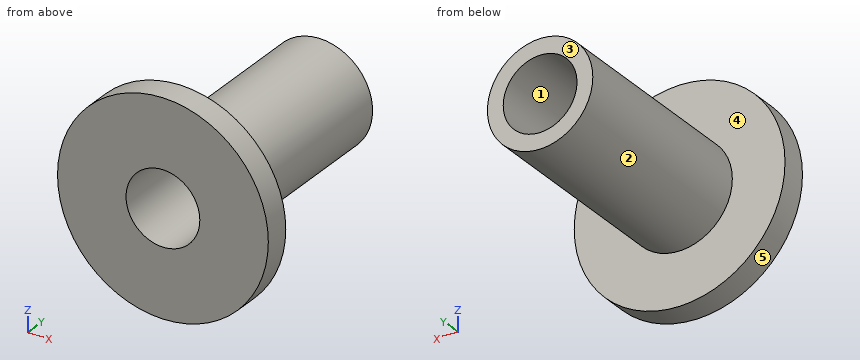
Autodesk Inventor part; units mm, degrees
ref_plane "YZ Plane" through (0, 0, 0) normal (1, 0, 0) x (0, 1, 0)
ref_plane "XZ Plane" through (0, 0, 0) normal (0, 1, 0) x (-1, 0, 0)
ref_plane "XY Plane" through (0, 0, 0) normal (0, 0, 1) x (1, 0, 0)
sketch "Sketch1" plane through (0, 0, 0) normal (0, 1, 0) x (-1, 0, 0)
  circle A0 centre (0, 0) radius 6.35
  dimension "d0" = 12.7
extrude "Extrusion1" add sketch "Sketch1" along normal blind 25.4
sketch "Sketch2" plane through (0, 25.4, 0) normal (0, 1, 0) x (1, 0, 0)
  circle A0 centre (0, 0) radius 4.445
  dimension "d3" = 8.89
extrude "Extrusion2" cut sketch "Sketch2" against normal blind 28.575
sketch "Sketch3" plane through (0, 0, 0) normal (0, -1, 0) x (1, 0, 0)
  circle A0 centre (0, 0) radius 12.7
  dimension "d6" = 25.4
extrude "Extrusion3" add sketch "Sketch3" along normal blind 3.175
sketch "Sketch4" plane through (0, -3.175, 0) normal (0, -1, 0) x (1, 0, 0)
  circle A0 centre (0, 0) radius 4.445
  dimension "d9" = 8.89
extrude "Extrusion4" cut sketch "Sketch4" against normal blind 3.175
properties part number "Nut"
Part model, mm, in its own coordinate system. Face numbers are marked on the shaded views. A direction names the side the tool comes from. Give positions to 0.01 mm unless a question says otherwise; leave off trailing zeros. Order: outer loops, then holes, each group sorted by start corner. A loop starts at its lowest first (then second) coordinate and runs counter-clockwise, first axis right, second up. Notation, with made-up numbers: M 6,43.5 L 60,43.5 A31 ccw 60,67.5 Z; hole C -18,12.25 d11. An arc over 180 degrees is marked long. Use a Markdown table: item, result. Add a question column.
(1) Saw through at D-D, the plane z = -9.25. Give the cut face in (x, y) (3 decimals), and give its area (3 significant figures).
(2) Saw through at A-A, the plane x = 0. Give the cut face in (y, z) (3 decimals), and give its area (3 significant figures).
(3) Probe line 1 along Z through (x, y) = (0.25, 22.25); line 2 along Y through (x, z) = (1.5, 10) (3 decimals); line 3 along X through (y, z) = (8.25, -3.5). List the from-to ranges inside material, lowest first. Write a range as [from, to].
(4) Mould opens along Z. For the marked faces 1, 2 and 3 say: +Z half, -Z half, draft (parallel to the pull), parting line (faces both ways), or undercut.
(5) Drop flat-ended pins along their axis: P1, Ø2, axis at y = 3.5, z = 8, coming from the -X side; P2, Ø4, axis at y = 10.5, z = -5.5, coming from the -X side; P3, Ø5, axis at x = 8, y = 11, coming from the +Z side; P4, Ø3, axis at x = -6, y = 7.5, coming from the +Z side. Give the stop position or say it passes through.
(6) Saw through at C-C, the plane y = 12. Give the cut face in (x, z) (3 decimals).
(7) Saw through at B-B, the plane z = 0. Give the cut face in (x, y) (3 decimals).
(8) 3-axis set-ups, long thin cutter, end or side, ignore diameter. For the marked faces 4 and 5: which of +Z, -Z, +X, -X, +Y, -Y reach the whole face in a straight line?
Answer key:
| question | item | result |
|---|---|---|
| 1 | outline | M -8.702,-3.175 L 8.702,-3.175 L 8.702,0 L -8.702,0 Z |
| 1 | area | 55.3 mm^2 |
| 2 | outline | M -3.175,-12.7 L 0,-12.7 L 0,-6.35 L 25.4,-6.35 L 25.4,-4.445 L -3.175,-4.445 Z; M -3.175,4.445 L 25.4,4.445 L 25.4,6.35 L 0,6.35 L 0,12.7 L -3.175,12.7 Z |
| 2 | area | 149 mm^2 |
| 3 | line 1 | [-6.35, -4.44], [4.44, 6.35] |
| 3 | line 2 | [-3.175, 0] |
| 3 | line 3 | [-5.3, -2.74], [2.74, 5.3] |
| 4 | face 1 | undercut |
| 4 | face 2 | parting line |
| 4 | face 3 | draft |
| 5 | P1 | through |
| 5 | P2 | x = -5.3 |
| 5 | P3 | z = 3.17 |
| 5 | P4 | z = 4.48 |
| 6 | outline | C 0,0 d12.7; hole C 0,0 d8.89 |
| 7 | outline | M -12.7,-3.175 L -4.445,-3.175 L -4.445,25.4 L -6.35,25.4 L -6.35,0 L -12.7,0 Z; M 4.445,-3.175 L 12.7,-3.175 L 12.7,0 L 6.35,0 L 6.35,25.4 L 4.445,25.4 Z |
| 8 | face 4 | +Y |
| 8 | face 5 | +Y, -Y |
